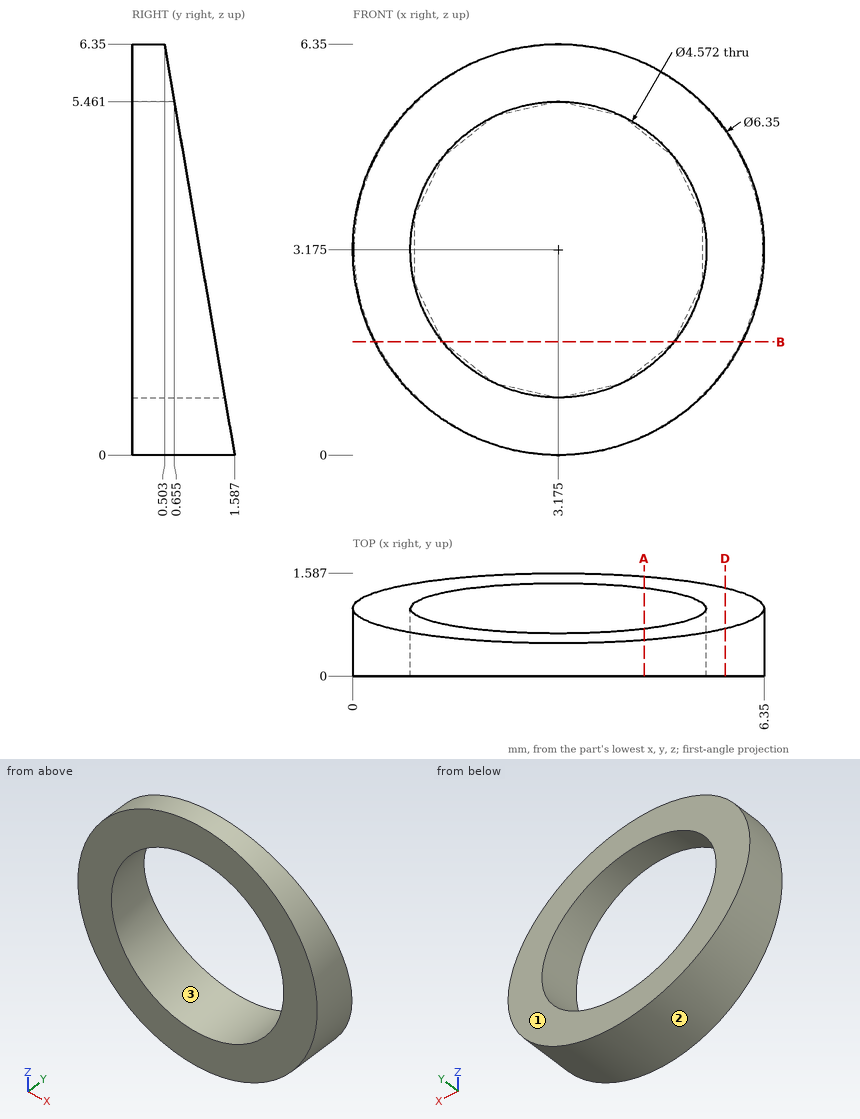
For this review, use the dimensioned drawing (mm, ordinates from the lowest corner) and the shaded views. Round coordinates to 2 decimals unless told otherwise and drop trailing zeros. Write each loop counter-clockwise with the first axis right and the second up, starting at its lowest first coordinate (ties: lowest second). Pieces come first, ordered by that corner, then holes. Notation, with made-up numbers: (-32.75, 39) -> (25.25, 39) arc R18 cw to (25.25, 43) -> close; hole circle Ø7 at (39, 72). An arc over 180 degrees is marked (long way). One line per item, written item: value. Start each with the question number.
Q1. Add section A-A (x = 4.5). Give the boundary of the cut face in (y, z).
Q2. Insertion check: P1, Ø2, axis at x = 2.5, z = 1, coming from the +Y side; P2, Ø3, axis at x = 1.5, z = 5.5, coming from the +Y side. Each pin has a flat end and moves straight along its axis. Give the tip position at first contact, or say it passes through.
Q3. Add section D-D (x = 5.75). Give the boundary of the cut face in (y, z).
Q4. Add section B-B (z = 1.75). Give the boundary of the cut face in (x, y).
Q5. To check wall thickness, follow probe 1 along X at (y, z) = (0.65, 3.25); probe 2 along X at (y, z) = (0.1, 4); probe 3 along Z at (x, y) = (4.25, 0.3). State the ranges of each line that lie inside material, in increasing order.
Q6. The part is to be moulded in two halves that separate along X. For the marked faces 1, 2 and 3, say which applies: pulls with the +X half, pulls with the -X half, needs draft (parallel to the pull), parting line crosses it, or undercut.
Response:
1. outline: (0, 0.29) -> (1.54, 0.29) -> (1.36, 1.31) -> (0, 1.31) -> close; (0, 5.04) -> (0.73, 5.04) -> (0.55, 6.06) -> (0, 6.06) -> close
2. P1: stops at y = 1.58
2. P2: stops at y = 0.89
3. outline: (0, 1.32) -> (1.36, 1.32) -> (0.73, 5.03) -> (0, 5.03) -> close
4. outline: (0.34, 0) -> (1.39, 0) -> (1.39, 1.29) -> (0.34, 1.29) -> close; (4.96, 0) -> (6.01, 0) -> (6.01, 1.29) -> (4.96, 1.29) -> close
5. probe 1: x = 0 to 0.89, 5.46 to 6.35
5. probe 2: x = 0.11 to 1.04, 5.31 to 6.24
5. probe 3: z = 0.19 to 1.16, 5.19 to 6.16
6. face 1: needs draft
6. face 2: parting line crosses it
6. face 3: undercut
